Design review of the part built by this model. Coordinates are the model's own, in mm. Round coordinates to 2 decimals unless told otherwise and drop trailing zeros. Loops run counter-clockwise (first coordinate to the right, second up) from the corner with the lowest first, then second, coordinate; pieces in that order, holes last. Notation, with made-up numbers: M 17,-20 L 49,-20 A20 cw 49,2 Z; hole C 1,29 d8. An arc over 180 degrees is marked long. One line per item, written item: value. Start each with the question number.
Item 1: We need section C-C (x = -44). Write out the cut boundary in (y, z), then the cut area to 3 significant figures.
Item 2: We need section B-B (y = 2.9). Write out the cut boundary in (x, z), then the cut area to 3 significant figures.
Item 3: For line 1 along Z through (x, y) = (-46, 5.2); line 2 along X through (y, z) = (0.3, -0.5); line 3 along X through (y, z) = (3.3, -27.5), list the stretches that pass through material, from the lowest coordinate up.
Item 4: We need section D-D (x = 0). Write out the cut boundary in (y, z), then the cut area to 3 significant figures.
Item 5: We need section A-A (z = 0). Write out the cut boundary in (x, y), then the cut area to 3 significant figures.
from build123d import *

# Parameters (mm, degrees)
SKETCH1_W                = 104
SKETCH1_H                = 86
SKETCH1_R                = 30
SKETCH1_W_2              = 12
SKETCH1_H_2              = 6.5
MOTOR_CRADLE_PLATE_DEPTH = 6


with BuildPart() as part:
    # Sketch1 → Motor_Cradle_Plate (new body)
    with BuildSketch(Plane(origin=(0, 0, 0), x_dir=(1, 0, 0), z_dir=(0, 1, 0))):
        Rectangle(SKETCH1_W, SKETCH1_H)
        with Locations(Location((0, 0, 0), (0, 0, 270))):
            Circle(SKETCH1_R, mode=Mode.SUBTRACT)
        with Locations((-44, -30)):
            Rectangle(SKETCH1_W_2, SKETCH1_H_2, mode=Mode.SUBTRACT)
        with Locations((-44, 30)):
            Rectangle(SKETCH1_W_2, SKETCH1_H_2, mode=Mode.SUBTRACT)
        with Locations((44, -30)):
            Rectangle(SKETCH1_W_2, SKETCH1_H_2, mode=Mode.SUBTRACT)
        with Locations((44, 30)):
            Rectangle(SKETCH1_W_2, SKETCH1_H_2, mode=Mode.SUBTRACT)
    extrude(amount=MOTOR_CRADLE_PLATE_DEPTH)


solid = part.part
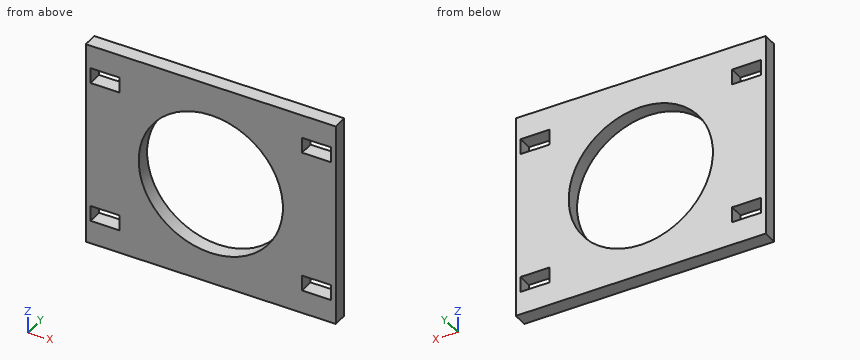
A:
1. outline: M 0,-43 L 6,-43 L 6,-33.25 L 0,-33.25 Z; M 0,-26.75 L 6,-26.75 L 6,26.75 L 0,26.75 Z; M 0,33.25 L 6,33.25 L 6,43 L 0,43 Z
1. area: 438 mm2
2. outline: M -52,-43 L 52,-43 L 52,43 L -52,43 Z; hole M -50,-33.25 L -38,-33.25 L -38,-26.75 L -50,-26.75 Z; hole M -50,26.75 L -38,26.75 L -38,33.25 L -50,33.25 Z; hole C 0,0 d60; hole M 38,-33.25 L 50,-33.25 L 50,-26.75 L 38,-26.75 Z; hole M 38,26.75 L 50,26.75 L 50,33.25 L 38,33.25 Z
2. area: 5,800 mm2
3. line 1: -43 to -33.25, -26.75 to 26.75, 33.25 to 43
3. line 2: -52 to -30, 30 to 52
3. line 3: -52 to -50, -38 to -11.99, 11.99 to 38, 50 to 52
4. outline: M 0,-43 L 6,-43 L 6,-30 L 0,-30 Z; M 0,30 L 6,30 L 6,43 L 0,43 Z
4. area: 156 mm2
5. outline: M -52,0 L -30,0 L -30,6 L -52,6 Z; M 30,0 L 52,0 L 52,6 L 30,6 Z
5. area: 264 mm2
